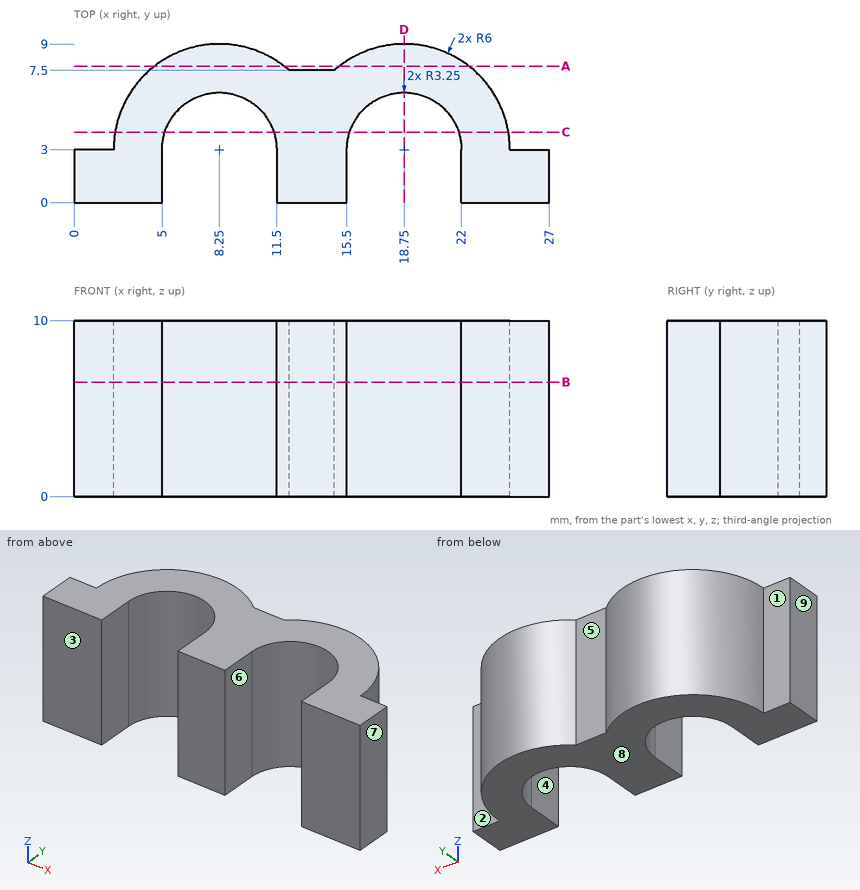
Here's the drawing with two shaded views (mm, measured from the low corner). I have some questions. A direction names the side the tool comes from. Round coordinates to 2 decimals unless told otherwise and drop trailing zeros. Write each loop counter-clockwise with the first axis right and the second up, starting at its lowest first coordinate (ties: lowest second). Pieces come first, ordered by that corner, then holes. Notation, with made-up numbers: M 63.5,4.25 L 104.5,4.25 A25 ccw 104.5,33.25 Z; hole C -29.5,5.25 d9. An arc over 180 degrees is marked long. Use CSV: the item, a comma, the result in double quotes.
(1) We'd pull the mould along X, two halves only. Please class the marked faces 6, 7, 8 and 9: +X half, -X half, draft (parallel to the pull), parting line (faces both ways), or undercut.
Check values:
face 6,"undercut"
face 7,"+X half"
face 8,"draft"
face 9,"-X half"
(2) Imagine slicing it at A-A (y = 7.75). Write out the boundary of the cut face in (x, z), plus the area to 3 significant figures.
Check values:
outline,"M 4.58,0 L 11.92,0 L 11.92,10 L 4.58,10 Z; M 15.08,0 L 22.42,0 L 22.42,10 L 15.08,10 Z"
area,"147 mm^2"
(3) I'm going to push flat-ended pins straight in: pin 1 (2.5 mm diameter, centred on x = 25.5, z = 6, fed in from +Y); pin 2 (1.5 mm diameter, centred on y = 1.5, z = 5.5, fed in from -X); pin 3 (1.8 mm diameter, centred on x = 1, z = 4, fed in from +Y); pin 4 (3 mm diameter, centred on y = 7, z = 2.5, fed in from -X). Where does each tip first touch, or does it pass through?
Check values:
pin 1,"y = 5.4"
pin 2,"x = 0"
pin 3,"y = 3"
pin 4,"x = 2.8"
(4) I need wall thicknesses on line 1 along X through (y, z) = (1, 3.5); line 2 along X through (y, z) = (4, 6); line 3 along Y through (x, z) = (18.75, 2). Which ranges of each line are inside material? Lowest first, please.
Check values:
line 1,"0 to 5, 11.5 to 15.5, 22 to 27"
line 2,"2.33 to 5.16, 11.34 to 15.66, 21.84 to 24.67"
line 3,"6.25 to 9"
(5) Imagine slicing it at C-C (y = 4). Write out the boundary of the cut face in (x, z), plus the area to 3 significant figures.
Check values:
outline,"M 2.33,0 L 5.16,0 L 5.16,10 L 2.33,10 Z; M 11.34,0 L 15.66,0 L 15.66,10 L 11.34,10 Z; M 21.84,0 L 24.67,0 L 24.67,10 L 21.84,10 Z"
area,"99.6 mm^2"
(6) Imagine slicing it at B-B (z = 6.5). Write out the boundary of the cut face in (x, y).
Check values:
outline,"M 0,0 L 5,0 L 5,3 A3.25 cw 11.5,3 L 11.5,0 L 15.5,0 L 15.5,3 A3.25 cw 22,3 L 22,0 L 27,0 L 27,3 L 24.75,3 A6 ccw 14.78,7.5 L 12.22,7.5 A6 ccw 2.25,3 L 0,3 Z"
(7) On a 3-axis mill with a long thin cutter (end or side, diameter ignored), from which of +Z, -Z, +X, -X, +Y, -Y can I reach the whole of each face in a straight line? I mean the marked faces 1, 2, 3, 4 and 5. Say none if no direction works.
Check values:
face 1,"+Z, -Z, -X, +Y"
face 2,"+Z, -Z, +X, +Y"
face 3,"+Z, -Z, +X, -X, -Y"
face 4,"+Z, -Z, -Y"
face 5,"+Z, -Z, +Y"
(8) Imagine slicing it at D-D (x = 18.75). Write out the boundary of the cut face in (y, z), plus the area to 3 significant figures.
Check values:
outline,"M 6.25,0 L 9,0 L 9,10 L 6.25,10 Z"
area,"27.5 mm^2"
